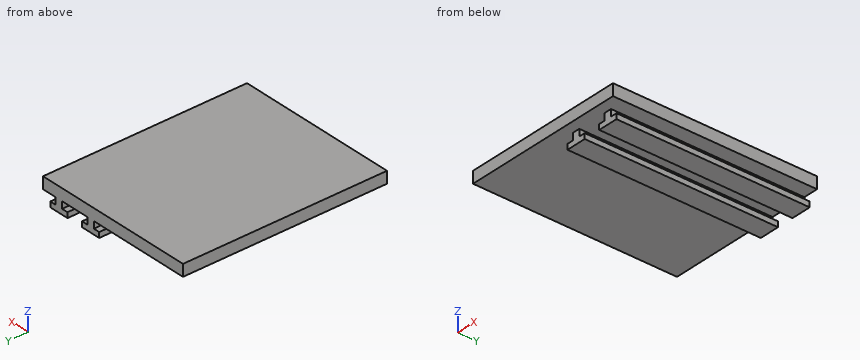
```python
from build123d import *

# Parameters (mm, degrees)
SKETCH_1_W          = 120
SKETCH_1_H          = 140
EXTRUDE_1_DEPTH     = 5.5
EXTRUDE_13_DEPTH    = 91
SKETCH_26_W         = 120
SKETCH_26_H         = 43.949941981
CUT_EXTRUDE_1_DEPTH = 10
SKETCH_27_W         = 42.806130355
SKETCH_27_H         = 96.050058019
CUT_EXTRUDE_2_DEPTH = 12.25


with BuildPart() as part:
    # 草图1 → 凸台-拉伸1 (new body)
    with BuildSketch(Plane.XY.offset(133)):
        with Locations((-63.049709027, -28.203400415)):
            Rectangle(SKETCH_1_W, SKETCH_1_H)
    extrude(amount=EXTRUDE_1_DEPTH)

    # 草图25 → 凸台-拉伸13 (add)
    with BuildSketch(Plane(origin=(0, 41.796599585, 0), x_dir=(1, 0, 0), z_dir=(0, 1, 0))):
        Polygon((-10.052220086, -133), (-10.052220086, -129.75), (-7.052220086, -129.75), (-7.052220086, -127.25), (-16.547197967, -127.25), (-16.547197967, -129.75), (-13.547197967, -129.75), (-13.547197967, -133), align=None)
        Polygon((-27.552220086, -133), (-27.552220086, -129.75), (-24.552220086, -129.75), (-24.552220086, -127.25), (-34.047197967, -127.25), (-34.047197967, -129.75), (-31.047197967, -129.75), (-31.047197967, -133), align=None)
    extrude(amount=-EXTRUDE_13_DEPTH)

    # 草图26 → 切除-拉伸1 (cut)
    with BuildSketch(Plane.XY.offset(138.5)):
        with Locations((-63.049709027, -76.228429425)):
            Rectangle(SKETCH_26_W, SKETCH_26_H)
    extrude(amount=-CUT_EXTRUDE_1_DEPTH, mode=Mode.SUBTRACT)

    # 草图27 → 切除-拉伸2 (cut, through all)
    with BuildSketch(Plane.XY.offset(138.5)):
        with Locations((-101.64664385, -6.228429424)):
            Rectangle(SKETCH_27_W, SKETCH_27_H)
    extrude(amount=-CUT_EXTRUDE_2_DEPTH, mode=Mode.SUBTRACT)


solid = part.part
```
Geometry: final body of the model. Coordinates: model frame, mm. Coordinates: 2 decimals unless noted, no trailing zeros. Order: outer loops, then holes, each group sorted by start corner. A loop starts at its lowest first (then second) coordinate and runs counter-clockwise, first axis right, second up. Notation, with made-up numbers: (-11, 83.25) -> (0, 83.25) arc R19 ccw to (0, 117.25) -> close; hole circle Ø9 at (-31.5, 26). An arc over 180 degrees is marked (long way). Write each question's results on one line, items separated by ' | '. Start each with the question number.
1) Cut plane B-B, the plane z = 132. Output: boundary loops of the cut face in (x, y).
2) Material intervals for line 1 along X through (y, z) = (-22, 132); line 2 along Z through (x, y) = (-32, -34.5); line 3 along Z through (x, y) = (-24, -48), sorted ascending.
3) Cut plane C-C, the plane y = 4.5. Output: boundary loops of the cut face in (x, z).
4) Cut plane D-D, the plane x = -38.5. Output: boundary loops of the cut face in (y, z).
5) Cut plane A-A, the plane x = -26.5. Output: boundary loops of the cut face in (y, z).
6) First-contact query: pin 1 (3 mm diameter, centred on y = -10, z = 128, fed in from -X); pin 2 (1.2 mm diameter, centred on y = -11.5, z = 129, fed in from +X); pin 3 (1 mm diameter, centred on x = -67, y = -10.5, fed in from -Z). Flat tips, straight axial feed; report the tip coordinate or a pass-through.
Checks:
1) outline: (-31.05, -49.2) -> (-27.55, -49.2) -> (-27.55, 41.8) -> (-31.05, 41.8) -> close; (-13.55, -49.2) -> (-10.05, -49.2) -> (-10.05, 41.8) -> (-13.55, 41.8) -> close
2) line 1: -31.05 to -27.55, -13.55 to -10.05 | line 2: 127.25 to 129.75, 133 to 138.5 | line 3: 133 to 138.5
3) outline: (-80.24, 133) -> (-31.05, 133) -> (-31.05, 129.75) -> (-34.05, 129.75) -> (-34.05, 127.25) -> (-24.55, 127.25) -> (-24.55, 129.75) -> (-27.55, 129.75) -> (-27.55, 133) -> (-13.55, 133) -> (-13.55, 129.75) -> (-16.55, 129.75) -> (-16.55, 127.25) -> (-7.05, 127.25) -> (-7.05, 129.75) -> (-10.05, 129.75) -> (-10.05, 133) -> (-3.05, 133) -> (-3.05, 138.5) -> (-80.24, 138.5) -> close
4) outline: (-54.25, 133) -> (41.8, 133) -> (41.8, 138.5) -> (-54.25, 138.5) -> close
5) outline: (-54.25, 133) -> (41.8, 133) -> (41.8, 138.5) -> (-54.25, 138.5) -> close; (-49.2, 127.25) -> (41.8, 127.25) -> (41.8, 129.75) -> (-49.2, 129.75) -> close
6) pin 1: x = -34.05 | pin 2: x = -7.05 | pin 3: z = 133
